```python
from build123d import *

# Parameters (mm, degrees)
SKETCH1_W              = 374.65
SKETCH1_H              = 295.275
BOSS_EXTRUDE1_DEPTH    = 3.175
FILLET1_R              = 12.7
SKETCH2_R              = 3.2639
SKETCH2_R_2            = 4.1021
CUT_EXTRUDE1_DEPTH     = 4.175
SKETCH3_W              = 28.448
SKETCH3_H              = 20.828
CUT_EXTRUDE2_DEPTH     = 4.175
F_4_40_TAPPED_HOLE1_D  = 2.2606
FILLET2_R              = 3.175
CUT_EXTRUDE3_DEPTH     = 4.175
SKETCH7_R              = 6.35
CUT_EXTRUDE4_DEPTH     = 4.175
F_10_32_TAPPED_HOLE_D  = 4.0386
F_8_32_TAPPED_HOLE1_D  = 3.4544
F_10_CLEARANCE_HOLE2_D = 5.1054


with BuildPart() as part:
    # Sketch1 → Boss-Extrude1 (new body)
    with BuildSketch(Plane(origin=(0, 0, 0), x_dir=(1, 0, 0), z_dir=(0, 1, 0))):
        Rectangle(SKETCH1_W, SKETCH1_H)
    extrude(amount=BOSS_EXTRUDE1_DEPTH)

    # Fillet1
    fillet1_edges = [part.edges().sort_by_distance(p)[0] for p in [
        (187.325, 1.5875, 147.6375),
        (-187.325, 1.5875, 147.6375),
        (-187.325, 1.5875, -147.6375),
        (187.325, 1.5875, -147.6375),
    ]]
    fillet(fillet1_edges, radius=FILLET1_R)

    # Sketch2 → Cut-Extrude1 (cut, through all)
    with BuildSketch(Plane(origin=(0, 3.175, 0), x_dir=(1, 0, 0), z_dir=(0, 1, 0))):
        with Locations((-22.252205122, 122.2375)):
            Circle(SKETCH2_R)
        with Locations((-22.252205122, 106.3625)):
            Circle(SKETCH2_R)
        with Locations((-22.252205122, 90.4875)):
            Circle(SKETCH2_R)
        with Locations((-22.252205122, 74.6125)):
            Circle(SKETCH2_R)
        with Locations((-22.252205122, 58.7375)):
            Circle(SKETCH2_R)
        with Locations((-22.252205122, 42.8625)):
            Circle(SKETCH2_R)
        with Locations((-22.252205122, 26.9875)):
            Circle(SKETCH2_R)
        with Locations((-22.252205122, 11.1125)):
            Circle(SKETCH2_R)
        with Locations((3.147794878, 122.2375)):
            Circle(SKETCH2_R_2)
        with Locations((3.147794878, 106.3625)):
            Circle(SKETCH2_R_2)
        with Locations((3.147794878, 90.4875)):
            Circle(SKETCH2_R_2)
        with Locations((3.147794878, 74.6125)):
            Circle(SKETCH2_R_2)
        with Locations((3.147794878, 58.7375)):
            Circle(SKETCH2_R_2)
        with Locations((3.147794878, 42.8625)):
            Circle(SKETCH2_R_2)
        with Locations((3.147794878, 26.9875)):
            Circle(SKETCH2_R_2)
        with Locations((3.147794878, 11.1125)):
            Circle(SKETCH2_R_2)
    extrude(amount=-CUT_EXTRUDE1_DEPTH, mode=Mode.SUBTRACT)

    # Sketch3 → Cut-Extrude2 (cut, through all)
    with BuildSketch(Plane(origin=(0, 3.175, 0), x_dir=(1, 0, 0), z_dir=(0, 1, 0))):
        with Locations((-154.6225, 124.5235)):
            Rectangle(SKETCH3_W, SKETCH3_H)
    extrude(amount=-CUT_EXTRUDE2_DEPTH, mode=Mode.SUBTRACT)

    # #4-40 Tapped Hole1 (through all)
    with Locations(Plane(origin=(0, 3.175, 0), x_dir=(1, 0, 0), z_dir=(0, 1, 0))):
        with Locations((-174.625, 124.5235), (-134.62, 124.5235)):
            Hole(F_4_40_TAPPED_HOLE1_D / 2)

    # Fillet2
    fillet2_edges = [part.edges().sort_by_distance(p)[0] for p in [
        (-140.3985, 1.5875, -134.9375),
        (-140.3985, 1.5875, -114.1095),
        (-168.8465, 1.5875, -114.1095),
        (-168.8465, 1.5875, -134.9375),
    ]]
    fillet(fillet2_edges, radius=FILLET2_R)

    # Sketch6 → Cut-Extrude3 (cut, through all)
    with BuildSketch(Plane(origin=(0, 3.175, 0), x_dir=(1, 0, 0), z_dir=(0, 1, 0))):
        with BuildLine():
            Line((-170.650952441, 100.965), (-165.899047559, 100.965))
            ThreePointArc((-165.899047559, 100.965), (-168.275, 92.075), (-170.650952441, 100.965))
        make_face()
        with BuildLine():
            Line((-151.600952441, 100.965), (-146.849047559, 100.965))
            ThreePointArc((-146.849047559, 100.965), (-149.225, 92.075), (-151.600952441, 100.965))
        make_face()
        with BuildLine():
            Line((-151.600952441, 81.915), (-146.849047559, 81.915))
            ThreePointArc((-146.849047559, 81.915), (-149.225, 73.025), (-151.600952441, 81.915))
        make_face()
    extrude(amount=-CUT_EXTRUDE3_DEPTH, mode=Mode.SUBTRACT)

    # Sketch7 → Cut-Extrude4 (cut, through all)
    with BuildSketch(Plane(origin=(0, 3.175, 0), x_dir=(1, 0, 0), z_dir=(0, 1, 0))):
        with Locations((-104.775, 122.2375)):
            Circle(SKETCH7_R)
    extrude(amount=-CUT_EXTRUDE4_DEPTH, mode=Mode.SUBTRACT)

    # #10-32 Tapped Hole (through all)
    with Locations(Plane(origin=(0, 3.175, 0), x_dir=(1, 0, 0), z_dir=(0, 1, 0))):
        with Locations((169.422510963, -25.341010963), (-12.847889037, -25.341010963), (-12.847889037, -129.735010963), (169.422510963, -129.735010963)):
            Hole(F_10_32_TAPPED_HOLE_D / 2)

    # #8-32 Tapped Hole1 (through all)
    with Locations(Plane(origin=(0, 3.175, 0), x_dir=(1, 0, 0), z_dir=(0, 1, 0))):
        with Locations((-117.585593705, -122.275595912), (-117.585593705, -71.475595912), (-45.50678376, -71.475595912), (-45.50678376, -122.275595912)):
            Hole(F_8_32_TAPPED_HOLE1_D / 2)

    # #10 Clearance Hole2 (through all)
    with Locations(Plane(origin=(0, 0, 0), x_dir=(-1, 0, 0), z_dir=(0, -1, 0))):
        with Locations((140.925, -8.702499665), (166.325, -8.702499665), (166.325, -40.452499665), (140.925, -40.452499665), (94.246188733, -40.452499665), (94.246188733, -8.702499665), (68.846188733, -8.702499665), (68.846188733, -40.452499665)):
            Hole(F_10_CLEARANCE_HOLE2_D / 2)


solid = part.part
```
Could you check a few things on this model? Use its own coordinates, in mm. Round coordinates to 2 decimals unless told otherwise and drop trailing zeros.
(1) Suppose I cut it at A-A on x = 3. State how many separate pieces and enclosed holes the cut face has, and give its area (3 significant figures).
Findings below:
separate pieces: 9
enclosed holes: 0
area: 729 mm2
(2) If I drill on probe 1 along X at (y, z) = (1.65, 40) (3 decimals); probe 2 along X at (y, z) = (0.95, -122.5) (1 decimal); probe 3 along Z at (x, y) = (-162, 1.9), over which ranges is the centre line in solid material (lowest first)?
Findings below:
probe 1: x = -187.325 to -168.837, -163.813 to -143.437, -138.413 to -96.758, -91.734 to -71.358, -66.334 to 187.325
probe 2: x = -187.3 to -168.8, -140.4 to -111.1, -98.4 to -25.5, -19 to -0.9, 7.2 to 187.3
probe 3: z = -147.64 to -134.94, -114.11 to 147.64
(3) Thinking about a two-plate mould opening in Z: for faces 1 (the face through (5.04, 1.61, -86.85)), 2 (the face through (-3, 3.175, -2)), 3 (the face through (183.506, 1.61, 144.016)), which applies, +Z half, -Z half, draft (parallel to the pull), parting line (faces both ways), or undercut?
Findings below:
face 1: undercut
face 2: draft
face 3: +Z half
